For this review, use the dimensioned drawing (mm, ordinates from the lowest corner) and the shaded views. Give positions to 0.01 mm unless a question says otherwise; leave off trailing zeros. Loops run counter-clockwise (first coordinate to the right, second up) from the corner with the lowest first, then second, coordinate; pieces in that order, holes last. Notation, with made-up numbers: M 86,25 L 120,25 A33 cw 120,63 Z; hole C -23,41.25 d2. An arc over 180 degrees is marked long. Use one line per item in the form item = value. Start each with the question number.
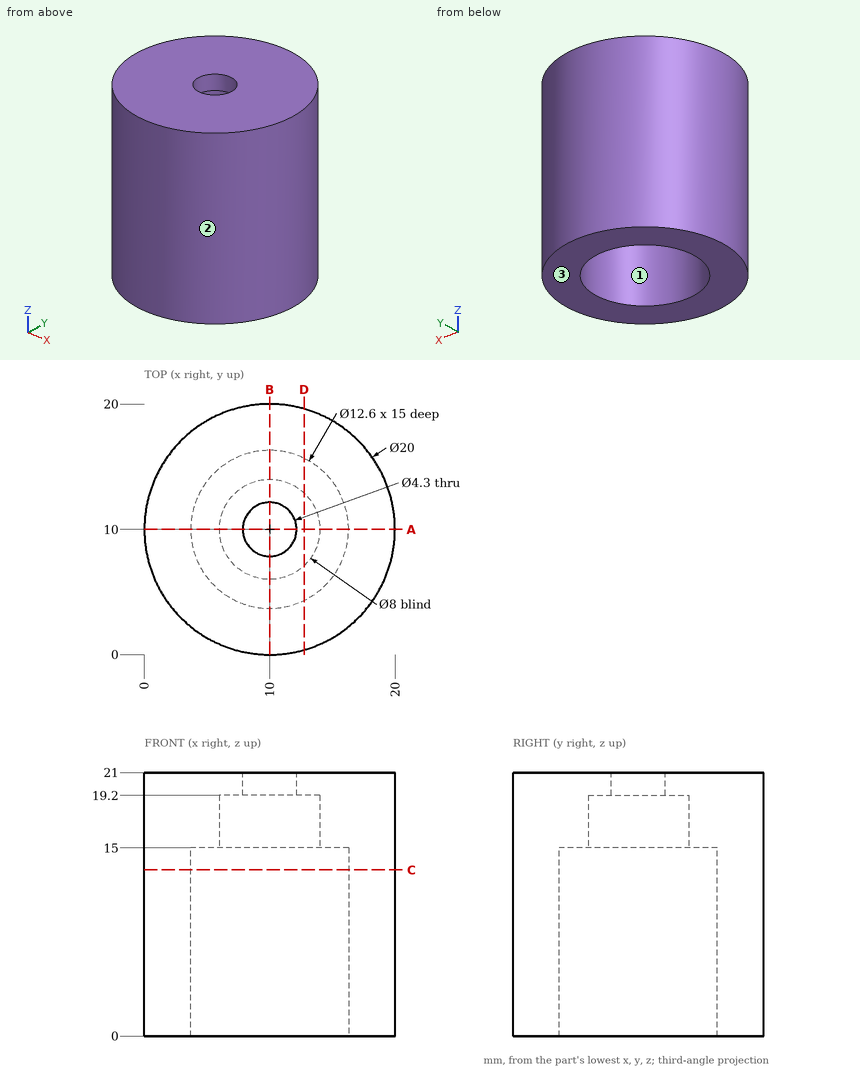
Q1. Take a section at D-D on x = 12.75. Give the boundary of the cut face in (y, z), plus the area to 3 significant figures.
Q2. The part is to be moulded in two halves that separate along Y. For the marked faces 1, 2 and 3, say which applies: pulls with the +Y half, pulls with the -Y half, needs draft (parallel to the pull), parting line crosses it, or undercut.
Q3. Wall thickness on probe 1 along Y at (x, z) = (10, 17.3); probe 2 along X at (y, z) = (10.25, 4.25): over which ranges is each line inside the solid? List them lowest first.
Q4. Take a section at C-C on z = 13.25. Give the boundary of the cut face in (x, y), plus the area to 3 significant figures.
Q5. Clearance check with flat-ended pins moving along their axes: pin 1 Ø2.5 at (x, y) = (10, 10) entering from -Z; pin 2 Ø6 at (y, z) = (6.5, 7) entering from +X; pin 3 Ø2.5 at (x, y) = (10.5, 8.5) entering from -Z; pin 4 Ø10 at (x, y) = (10, 10) entering from -Z. State where each tip first meets the part, or that it passes through.
Q6. Take a section at A-A on y = 10. Give the boundary of the cut face in (x, z), plus the area to 3 significant figures.
Response values:
q1.outline = M 0.39,0 L 4.33,0 L 4.33,15 L 7.1,15 L 7.1,19.2 L 12.9,19.2 L 12.9,15 L 15.67,15 L 15.67,0 L 19.61,0 L 19.61,21 L 0.39,21 Z
q1.area = 209 mm^2
q2.face_1 = undercut
q2.face_2 = parting line crosses it
q2.face_3 = needs draft
q3.probe_1 = 0 to 6, 14 to 20
q3.probe_2 = 0 to 3.7, 16.3 to 20
q4.outline = C 10,10 d20; hole C 10,10 d12.6
q4.area = 189 mm^2
q5.pin_1 = through
q5.pin_2 = 19.99
q5.pin_3 = 19.2
q5.pin_4 = 15
q6.outline = M 0,0 L 3.7,0 L 3.7,15 L 6,15 L 6,19.2 L 7.85,19.2 L 7.85,21 L 0,21 Z; M 12.15,19.2 L 14,19.2 L 14,15 L 16.3,15 L 16.3,0 L 20,0 L 20,21 L 12.15,21 Z
q6.area = 190 mm^2
